Check sheet for the drawn part. Datum: minimum x, y, z corner. Units: mm. Give positions to 0.01 mm unless a question says otherwise; leave off trailing zeros. Order: outer loops, then holes, each group sorted by start corner. A loop starts at its lowest first (then second) coordinate and runs counter-clockwise, first axis right, second up. Notation, with made-up numbers: (82.25, 19) - (106.25, 19) arc R19 cw to (106.25, 24) - close; hole circle Ø10 at (-6.75, -30.75). An arc over 180 degrees is marked (long way). Answer as a JSON object with one key per item and string values. Group by question number.
(1) Section check A-A (y = 15). Record the boundary of the cut face in (x, z), then the cut area to 3 significant figures.
(2) Section check B-B (x = 15). Record the boundary of the cut face in (y, z), then the cut area to 3 significant figures.
(3) Mould release check, pull along X, two halves, no side actions. Record for the marked faces 1, 2 and 3: +X half, -X half, draft (parallel to the pull), parting line (faces both ways), or undercut.
(4) Depth check by flat-ended pin: pin 1 Ø1.5 at (x, y) = (3.5, 38.5) entering from +Z; pin 2 Ø1.6 at (y, z) = (24, 8) entering from -X; pin 3 Ø0.8 at (x, z) = (25, 7.5) entering from -Y. Enter the tip coordinate at first touch or a pass-through.
(5) Thickness scan on line 1 (Y direction, x = 15, z = 4); line 2 (Y direction, x = 14.25, z = 2.5); line 3 (Z direction, x = 24.5, y = 19). Record the ranges inside material, lowest first.
(6) Section check D-D (y = 6.5). Record the boundary of the cut face in (x, z), then the cut area to 3 significant figures.
(7) Section check C-C (z = 5.5). Record the boundary of the cut face in (x, y).
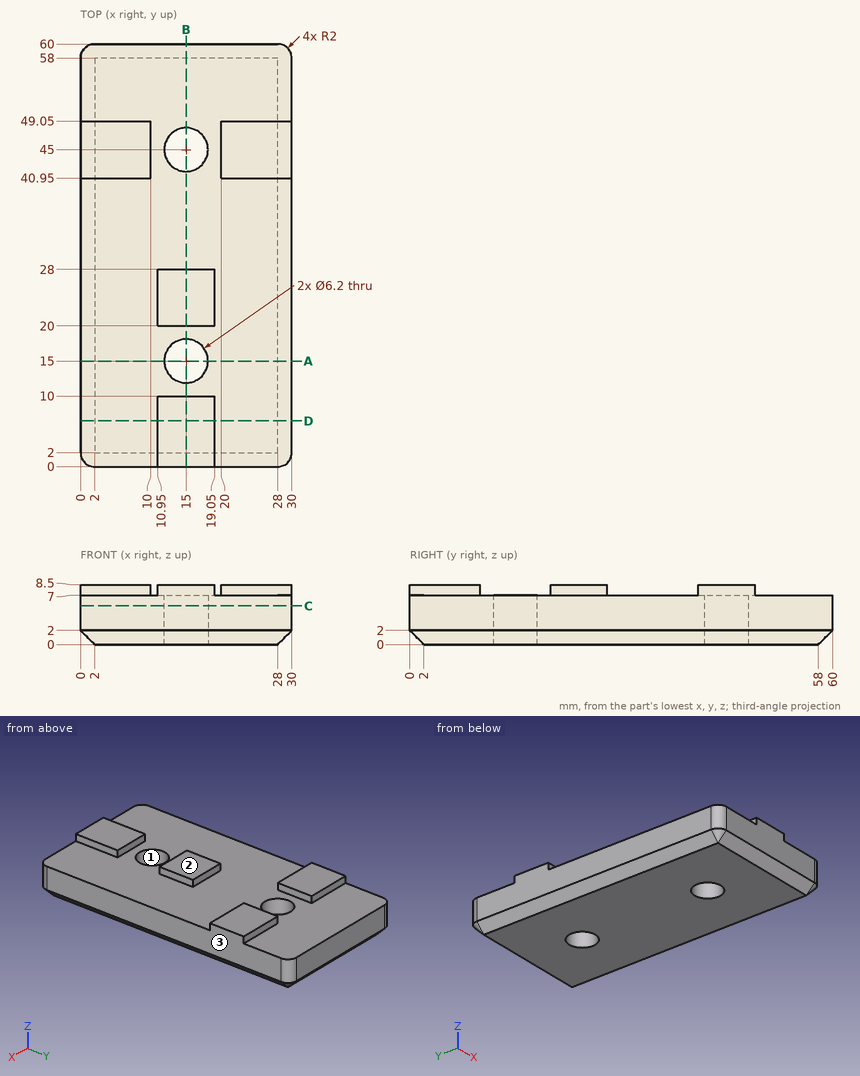
Solutions:
{
 "1": {"outline": "(0, 2) - (2, 0) - (11.9, 0) - (11.9, 7) - (0, 7) - close; (18.1, 0) - (28, 0) - (30, 2) - (30, 7) - (18.1, 7) - close", "area": "163 mm2"},
 "2": {"outline": "(0, 2) - (2, 0) - (11.9, 0) - (11.9, 7) - (10, 7) - (10, 8.5) - (0, 8.5) - close; (18.1, 0) - (41.9, 0) - (41.9, 7) - (28, 7) - (28, 8.5) - (20, 8.5) - (20, 7) - (18.1, 7) - close; (48.1, 0) - (58, 0) - (60, 2) - (60, 7) - (48.1, 7) - close", "area": "356 mm2"},
 "3": {"face 1": "undercut", "face 2": "draft", "face 3": "+X half"},
 "4": {"pin 1": "stops at z = 7", "pin 2": "stops at x = 10.95", "pin 3": "stops at y = 40.95"},
 "5": {"line 1": "y = 0 to 11.9, 18.1 to 41.9, 48.1 to 60", "line 2": "y = 0 to 11.99, 18.01 to 41.99, 48.01 to 60", "line 3": "z = 0 to 7"},
 "6": {"outline": "(0, 2) - (2, 0) - (28, 0) - (30, 2) - (30, 7) - (19.05, 7) - (19.05, 8.5) - (10.95, 8.5) - (10.95, 7) - (0, 7) - close", "area": "218 mm2"},
 "7": {"outline": "(0, 2) arc R2 ccw to (2, 0) - (28, 0) arc R2 ccw to (30, 2) - (30, 58) arc R2 ccw to (28, 60) - (2, 60) arc R2 ccw to (0, 58) - close; hole circle Ø6.2 at (15, 15); hole circle Ø6.2 at (15, 45)"}
}
